The model under review builds one solid part; all positions refer to its coordinate system, in mm. Round coordinates to 2 decimals unless told otherwise and drop trailing zeros. Loops run counter-clockwise (first coordinate to the right, second up) from the corner with the lowest first, then second, coordinate; pieces in that order, holes last. Notation, with made-up numbers: M -23,5.25 L 35,5.25 A18 ccw 35,23.25 Z; hole C -4,-14.5 d1. An arc over 180 degrees is marked long. Use a Markdown table: item, result. Add a question column.
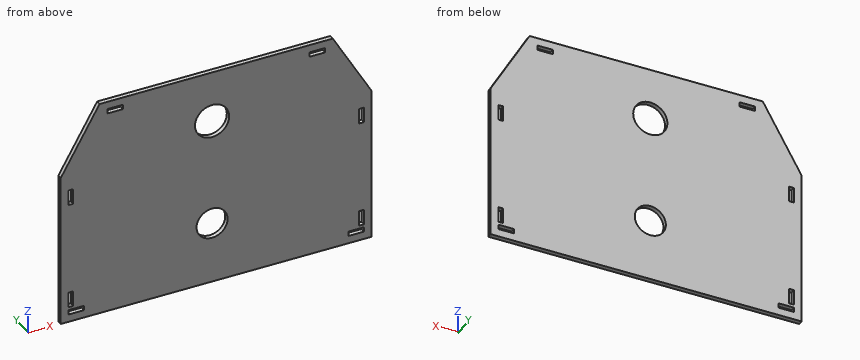
```python
from build123d import *

# Parameters (mm, degrees)
RESSALTO_EXTRUS_O1_DEPTH = 3
ESBO_O3_W                = 10
ESBO_O3_H                = 3
ESBO_O3_W_2              = 3
ESBO_O3_H_2              = 10
ESBO_O3_W_3              = 3.017337907
CORTE_EXTRUS_O1_DEPTH    = 3
ESBO_O5_R                = 10
ESBO_O5_R_2              = 11
CORTE_EXTRUS_O2_DEPTH    = 10


with BuildPart() as part:
    # Esboço1 → Ressalto-extrusão1 (new body)
    with BuildSketch(Plane(origin=(0, 0, 0), x_dir=(1, 0, 0), z_dir=(0, 1, 0))):
        Polygon((-97.357643635, -26.698729811), (-97.357643635, 73.301270189), (102.642356365, 73.301270189), (102.642356365, -26.698729811), (77.642356365, -70), (-72.357643635, -70), align=None)
    extrude(amount=RESSALTO_EXTRUS_O1_DEPTH)

    # Esboço3 → Corte-extrusão1 (cut)
    with BuildSketch(Plane(origin=(0, 3, 0), x_dir=(1, 0, 0), z_dir=(0, 1, 0))):
        with Locations((-62.357643635, -63.5)):
            Rectangle(ESBO_O3_W, ESBO_O3_H)
        with Locations((67.642356365, -63.5)):
            Rectangle(ESBO_O3_W, ESBO_O3_H)
        with Locations((96.142356365, -11.698729811)):
            Rectangle(ESBO_O3_W_2, ESBO_O3_H_2)
        with Locations((96.133687412, 58.301270189)):
            Rectangle(ESBO_O3_W_3, ESBO_O3_H_2)
        with Locations((92.642356365, 66.801270189)):
            Rectangle(ESBO_O3_W, ESBO_O3_H)
        with Locations((-90.857643635, -11.698729811)):
            Rectangle(ESBO_O3_W_2, ESBO_O3_H_2)
        with Locations((-90.857643635, 58.301270189)):
            Rectangle(ESBO_O3_W_2, ESBO_O3_H_2)
        with Locations((-87.357643635, 66.801270189)):
            Rectangle(ESBO_O3_W, ESBO_O3_H)
    extrude(amount=-CORTE_EXTRUS_O1_DEPTH, mode=Mode.SUBTRACT)

    # Esboço5 → Corte-extrusão2 (cut)
    with BuildSketch(Plane(origin=(0, 3, 0), x_dir=(1, 0, 0), z_dir=(0, 1, 0))):
        with Locations(Location((0, 33.301270189, 0), (0, 0, 270))):
            Circle(ESBO_O5_R)
        with Locations(Location((0, -36.698729811, 0), (0, 0, 270))):
            Circle(ESBO_O5_R_2)
    extrude(amount=-CORTE_EXTRUS_O2_DEPTH, mode=Mode.SUBTRACT)


solid = part.part
```
(1) Consider section A-A, the plane x = 0. Give the boundary of the cut face in (y, z).
(2) Insertion check: pin 1 Ø5 at (x, z) = (-20.5, 21.5) entering from -Y; pin 2 Ø0.9 at (x, y) = (95.5, 2) entering from +Z; pin 3 Ø1.5 at (y, z) = (2, 63) entering from -X. Each pin has a flat end and moves straight along its axis. Give the tip position at first contact, or say it passes through.
(3) Consider section B-B, the plane y = 1.2. Give the number of separate pieces and of enclosed holes in the cut face, then the cut area to 3 significant figures.
(4) To check wall thickness, follow probe 1 along X at (y, z) = (2.1, -56); probe 2 along Z at (x, y) = (-1, 0.9); probe 3 along X at (y, z) = (2.15, 40.5). State the ranges of each line that lie inside material, in increasing order.
Found:
| question | item | result |
|---|---|---|
| 1 | outline | M 0,-73.3 L 3,-73.3 L 3,-43.3 L 0,-43.3 Z; M 0,-23.3 L 3,-23.3 L 3,25.7 L 0,25.7 Z; M 0,47.7 L 3,47.7 L 3,70 L 0,70 Z |
| 2 | pin 1 | stops at y = 0 |
| 2 | pin 2 | stops at z = 39.85 |
| 2 | pin 3 | stops at x = -76.83 |
| 3 | separate pieces | 1 |
| 3 | enclosed holes | 10 |
| 3 | area | 26,600 mm^2 |
| 4 | probe 1 | x = -97.36 to -92.36, -89.36 to 94.63, 97.64 to 102.64 |
| 4 | probe 2 | z = -73.3 to -43.25, -23.35 to 25.74, 47.65 to 70 |
| 4 | probe 3 | x = -89.39 to -10.32, 10.32 to 94.67 |
